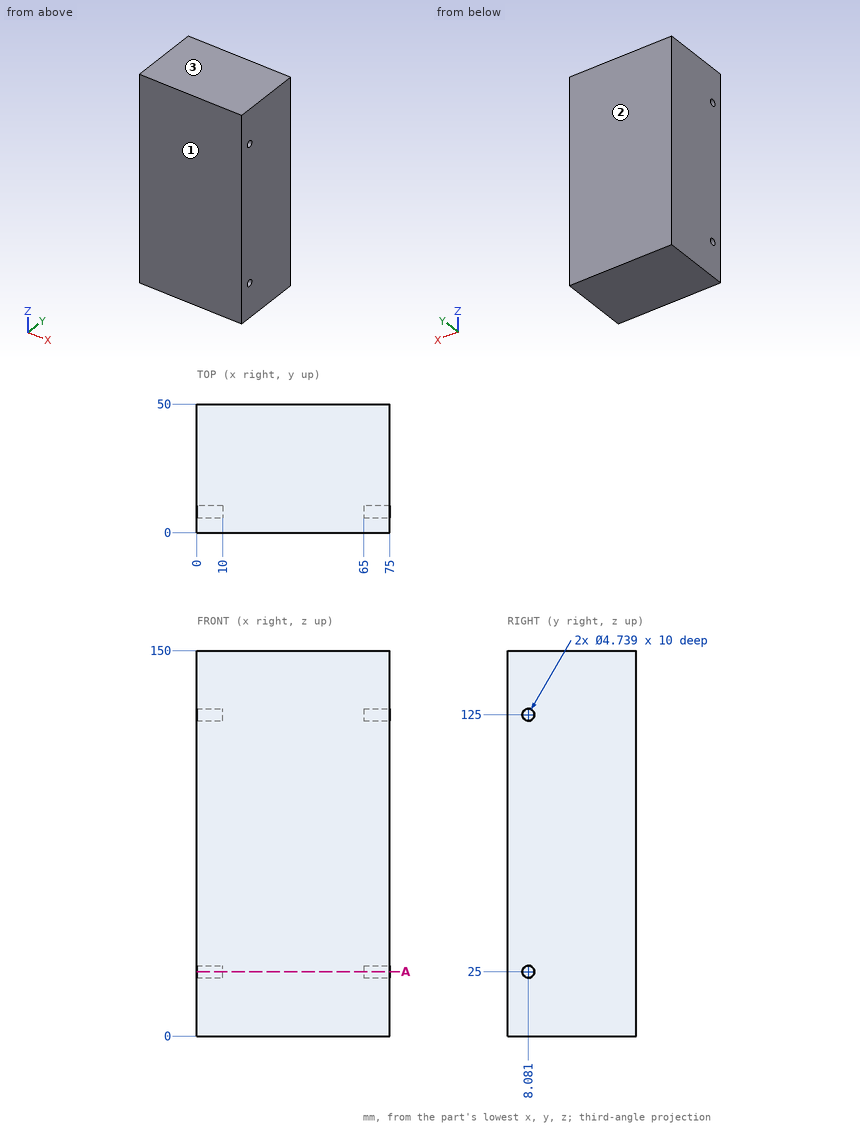
Job drawing, mm, ordinate dimensions from the low corner. One solid piece. Coordinates: 2 decimals unless noted, no trailing zeros. Order: outer loops, then holes, each group sorted by start corner. A loop starts at its lowest first (then second) coordinate and runs counter-clockwise, first axis right, second up. Notation, with made-up numbers: (85, -31) -> (93, -31) arc R33 ccw to (93, 0) -> close; hole circle Ø2 at (25.5, 59). An arc over 180 degrees is marked (long way). Answer in a Markdown table with one row per item. Add a question column.
Q1. Mould opens along Y. For the marked faces 1, 2 and 3 say: +Y half, -Y half, draft (parallel to the pull), parting line (faces both ways), or undercut.
Q2. Band-saw the part on A-A, the plane z = 25. List the corners of the cut face in (x, y).
Q3. Drop flat-ended pins along their axis: pin 1 (3 mm diameter, centred on y = 8.08, z = 25, fed in from +X); pin 2 (1.4 mm diameter, centred on y = 7.5, z = 124, fed in from -X). Give the stop position or say it passes through.
Q4. Wall check: line 1 along Y through (x, z) = (7.5, 125). Give the ranges that are in metal, low to high. Write a range as [from, to].
Answers follow:
| question | item | result |
|---|---|---|
| 1 | face 1 | -Y half |
| 1 | face 2 | +Y half |
| 1 | face 3 | draft |
| 2 | outline | (0, 0) -> (75, 0) -> (75, 5.71) -> (65, 5.71) -> (65, 10.45) -> (75, 10.45) -> (75, 50) -> (0, 50) -> (0, 10.45) -> (10, 10.45) -> (10, 5.71) -> (0, 5.71) -> close |
| 3 | pin 1 | x = 65 |
| 3 | pin 2 | x = 10 |
| 4 | line 1 | [0, 5.71], [10.45, 50] |
